from build123d import *

# Parameters (mm, degrees)
F0_W         = 100
F0_H         = 10
F1_DEPTH     = 51
F2_DEPTH     = 26
F3_DEPTH     = 29
F4_R         = 5
F5_W         = 100
F5_H         = 3
F6_DEPTH     = 2
F7_T4_DEPTH  = 115.4300979278
F8_W         = 100
F8_H         = 3
F9_DEPTH     = 2
F10_T4_DEPTH = 115.4300979278
F11_R        = 1


# Not quite as in the source:
# - a fillet or chamfer that OpenCascade refuses, or shapes differently, is made with other operations: its cross-section is extruded or revolved along the edge and cut away or added


with BuildPart() as f1:
    # F0 (on Top) → F1 (new body)
    with BuildSketch(Plane.XY):
        with Locations((50, -5)):
            Rectangle(F0_W, F0_H)
    extrude(amount=F1_DEPTH)



with BuildPart() as f1b:
    # F0 (on Top) → F1, piece 2 (new body)
    with BuildSketch(Plane.XY):
        with Locations((50, -56)):
            Rectangle(F0_W, F0_H)
    extrude(amount=F1_DEPTH)


with BuildPart() as f1_1:
    add(f1.part)

    add(f1b.part)  # F2 merges F1b
    # F0 (on Top) → F2 (join)
    with BuildSketch(Plane.XY):
        with Locations((50, -5)):
            Rectangle(F0_W, F0_H)
        with BuildLine():
            Line((100, -10), (0, -10))
            Line((0, -10), (0, -30.5))
            Line((0, -30.5), (46, -30.5))
            ThreePointArc((46, -30.5), (50, -26.5), (54, -30.5))
            Line((54, -30.5), (100, -30.5))
            Line((100, -30.5), (100, -10))
        make_face()
        with BuildLine():
            Line((46, -30.5), (0, -30.5))
            Line((0, -30.5), (0, -51))
            Line((0, -51), (100, -51))
            Line((100, -51), (100, -30.5))
            Line((100, -30.5), (54, -30.5))
            ThreePointArc((54, -30.5), (50, -34.5), (46, -30.5))
        make_face()
        with Locations((50, -56)):
            Rectangle(F0_W, F0_H)
        with BuildLine():
            ThreePointArc((54, -30.5), (50, -26.5), (46, -30.5))
            Line((46, -30.5), (49, -30.5))
            ThreePointArc((49, -30.5), (50, -29.5), (51, -30.5))
            Line((51, -30.5), (54, -30.5))
        make_face()
        with BuildLine():
            Line((49, -30.5), (46, -30.5))
            ThreePointArc((46, -30.5), (50, -34.5), (54, -30.5))
            Line((54, -30.5), (51, -30.5))
            ThreePointArc((51, -30.5), (50, -31.5), (49, -30.5))
        make_face()
    extrude(amount=F2_DEPTH)

    # F0 (on Top) → F3 (join)
    with BuildSketch(Plane.XY):
        with BuildLine():
            ThreePointArc((54, -30.5), (50, -26.5), (46, -30.5))
            Line((46, -30.5), (49, -30.5))
            ThreePointArc((49, -30.5), (50, -29.5), (51, -30.5))
            Line((51, -30.5), (54, -30.5))
        make_face()
        with BuildLine():
            Line((49, -30.5), (46, -30.5))
            ThreePointArc((46, -30.5), (50, -34.5), (54, -30.5))
            Line((54, -30.5), (51, -30.5))
            ThreePointArc((51, -30.5), (50, -31.5), (49, -30.5))
        make_face()
    extrude(amount=F3_DEPTH)

    # F4
    f4_edges = [f1_1.edges().sort_by_distance(p)[0] for p in [
        (100, 0, 25.5),
        (0, 0, 25.5),
        (100, -61, 25.5),
        (0, -61, 25.5),
    ]]
    fillet(f4_edges, radius=F4_R)

    # F5 (on face) → F6 (join)
    with BuildSketch(Plane.XY.offset(51)):
        with Locations((50, -11.5)):
            Rectangle(F5_W, F5_H)
    extrude(amount=-F6_DEPTH)

    # F7: chamfer of 3 on 1 edges, made by hand


with BuildPart() as f7_tool2:
    # F7_s3 → F7_t4 (new body)
    with BuildSketch(Plane.YZ.offset(-7.7150489639)):
        Polygon((-10, 49), (-13, 52), (-13, 49), align=None)
    extrude(amount=F7_T4_DEPTH)

    split(bisect_by=Plane.XZ.offset(10), keep=Keep.TOP)


with BuildPart() as f1_2:
    add(f1_1.part)

    # F7_t1: cut F7_tool2
    add(f7_tool2.part, mode=Mode.SUBTRACT)

    # F8 (on face) → F9 (join)
    with BuildSketch(Plane.XY.offset(51)):
        with Locations((50, -49.5)):
            Rectangle(F8_W, F8_H)
    extrude(amount=-F9_DEPTH)

    # F10: chamfer of 3 on 1 edges, made by hand


with BuildPart() as f10_tool2:
    # F10_s3 → F10_t4 (new body)
    with BuildSketch(Plane.YZ.offset(107.7150489639)):
        Polygon((-51, 49), (-48, 52), (-48, 49), align=None)
    extrude(amount=-F10_T4_DEPTH)

    split(bisect_by=Plane.XZ.offset(51), keep=Keep.BOTTOM)


with BuildPart() as f1_3:
    add(f1_2.part)

    # F10_t1: cut F10_tool2
    add(f10_tool2.part, mode=Mode.SUBTRACT)

    # F11
    f11_edges = [f1_3.edges().sort_by_distance(p)[0] for p in [
        (50, -12, 51),
        (50, -49, 51),
    ]]
    fillet(f11_edges, radius=F11_R)


solid = f1_3.part
Work out the finished part from the listing and answer in its coordinate system (mm). A direction names the side the tool comes from. Round coordinates to 2 decimals unless told otherwise and drop trailing zeros. Order: outer loops, then holes, each group sorted by start corner. A loop starts at its lowest first (then second) coordinate and runs counter-clockwise, first axis right, second up. Notation, with made-up numbers: M 6,14.5 L 45,14.5 A12 cw 45,29.5 Z; hole C 65.5,10.25 d9. An arc over 180 degrees is marked long. Put each result on its own line as item: value. Start each with the question number.
Q1. Flat-ended cylindrical pins translate along their axes: pin 1 (1 mm diameter, centred on x = 16, y = -36, fed in from +Z); pin 2 (4 mm diameter, centred on x = 51.5, y = -30.5, fed in from +Z). Find the tip coordinate at first contact, or state that the pin passes through.
Q2. Section B-B, the plane x = 34.5 is taken. Write down the section's boundary in (y, z).
Q3. For a pull along Y with two mould halves and no side action, classify faces 6 (the cylindrical face through (2, -1, 25)), 7 (the flat face through (49, -23, 0)), 8 (the cylindrical face through (2, -60, 26)), 9 (the flat face through (49, -26, 26)) as pulls with the +Y half, pulls with the -Y half, needs draft (parallel to the pull), parting line crosses it, or undercut.
Q4. Section A-A, the plane z = 47 is taken. Write down the section's boundary in (x, y), and give its area (3 significant figures).
Q5. Section C-C, the plane y = -24 is taken. Write down the section's boundary in (x, z).
Q6. A tool of negligible diameter and unlimited length cuts with its end or side. For faces 1 (the flat face through (49, -56, 51)), 2 (the cylindrical face through (52.95, -33.2, 27.48)), 3 (the flat face through (50.83, -31.33, 29)), 4 (the flat face through (49, -10, 37)), 5 (the cylindrical face through (99, -59, 25)), from which of +Z, -Z, +X, -X, +Y, -Y can it reach the whole face along a straight path? Write none if from no direction.
Q7. Straight lines are drawn through the part: L1, parallel to Y at x = 87, z = 44; L2, parallel to X at y = -30.5, z = 20; L3, parallel to Y at x = 50, z = 7.5. For each, find the intervals that lie inside material, in ascending order. Write a range as [from, to].
Findings below:
1. pin 1: stops at z = 26
1. pin 2: stops at z = 29
2. outline: M -61,0 L 0,0 L 0,51 L -9.59,51 A1 ccw -10.29,49.29 L -10,49 L -10,26 L -51,26 L -51,49 L -50.71,49.29 A1 ccw -51.41,51 L -61,51 Z
3. face 6: pulls with the +Y half
3. face 7: needs draft
3. face 8: pulls with the -Y half
3. face 9: undercut
4. outline: M 0,-56 A5 ccw 5,-61 L 95,-61 A5 ccw 100,-56 L 100,-51 L 0,-51 Z; M 0,-10 L 100,-10 L 100,-5 A5 ccw 95,0 L 5,0 A5 ccw 0,-5 Z
4. area: 1,980 mm^2
5. outline: M 0,0 L 100,0 L 100,26 L 0,26 Z
6. face 1: +Z, +X, -X, +Y, -Y
6. face 2: +Z
6. face 3: +Z, +X, -X
6. face 4: +X, -X
6. face 5: +Z, -Z, +X, -Y
7. L1: y = [-61, -51], [-10, 0]
7. L2: x = [0, 49], [51, 100]
7. L3: y = [-61, -31.5], [-29.5, 0]
